```python
from build123d import *

# Parameters (mm, degrees)
SKETCH1_W           = 43.18
SKETCH1_H           = 17.78
BOSS_EXTRUDE1_DEPTH = 12.7
CUT_EXTRUDE1_DEPTH  = 7.62
CUT_EXTRUDE2_DEPTH  = 18.78


with BuildPart() as part:
    # Sketch1 → Boss-Extrude1 (new body)
    with BuildSketch(Plane.XY):
        with Locations((21.59, 8.89)):
            Rectangle(SKETCH1_W, SKETCH1_H)
    extrude(amount=-BOSS_EXTRUDE1_DEPTH)

    # Sketch3 → Cut-Extrude1 (cut)
    with BuildSketch(Plane(origin=(0, 17.78, 0), x_dir=(1, 0, 0), z_dir=(0, 1, 0))):
        Polygon((43.18, 12.7), (36.83, 6.35), (43.18, 0), align=None)
    extrude(amount=-CUT_EXTRUDE1_DEPTH, mode=Mode.SUBTRACT)

    # Sketch4 → Cut-Extrude2 (cut, through all)
    with BuildSketch(Plane(origin=(0, 17.78, 0), x_dir=(1, 0, 0), z_dir=(0, 1, 0))):
        with BuildLine():
            Line((32.381000008, 4.599999944), (24.260999992, 4.599999944))
            ThreePointArc((24.260999992, 4.599999944), (22.510999936, 6.35), (24.260999992, 8.100000056))
            Line((24.260999992, 8.100000056), (32.381000008, 8.100000056))
            ThreePointArc((32.381000008, 8.100000056), (34.131000064, 6.35), (32.381000008, 4.599999944))
        make_face()
        with BuildLine():
            Line((15.68099988, 4.599999944), (7.560999864, 4.599999944))
            ThreePointArc((7.560999864, 4.599999944), (5.810999808, 6.35), (7.560999864, 8.100000056))
            Line((7.560999864, 8.100000056), (15.68099988, 8.100000056))
            ThreePointArc((15.68099988, 8.100000056), (17.430999936, 6.35), (15.68099988, 4.599999944))
        make_face()
    extrude(amount=-CUT_EXTRUDE2_DEPTH, mode=Mode.SUBTRACT)


solid = part.part
```
Design review of the part built by this model. Coordinates are the model's own, in mm. A direction names the side the tool comes from. Coordinates: 2 decimals unless noted, no trailing zeros. Order: outer loops, then holes, each group sorted by start corner. A loop starts at its lowest first (then second) coordinate and runs counter-clockwise, first axis right, second up. Notation, with made-up numbers: M 58.25,46 L 72.25,46 A15 ccw 72.25,74 Z; hole C -19.75,19 d3. An arc over 180 degrees is marked long. Answer as a JSON object with one key per item and string values. Group by question number.
1) Mouldability with a two-part tool opening along X and no side actions: class faces 1 (the flat face through (0, 9, -6)), 2 (the flat face through (12, 9, -4.6)), 3 (the flat face through (41, 10.16, -6)), 4 (the flat face through (40.05, 14.02, -9.57)) as pulls with the +X half, pulls with the -X half, needs draft (parallel to the pull), parting line crosses it, or undercut.
2) Wall thickness on L1, parallel to Z at x = 11.5, y = 8.25; L2, parallel to X at y = 10.25, z = -7.5; L3, parallel to X at y = 10.75, z = -5.25: over which ranges is each line inside the solid? List them lowest first.
3) Tool access review of faces 5 (the flat face through (21, 17.78, -6)), 6 (the flat face through (39.96, 14.02, -3.22)), 7 (the flat face through (28, 9, -4.6)): name each direction out of +Z, -Z, +X, -X, +Y, -Y from which nothing blocks a thin tool from reaching the whole face with its end or side.
4) For pin 1 (6 mm diameter, centred on y = 14, z = -10.5, fed in from +X), flat-tipped, find the tip position at first contact; note if it passes through.
5) Add section A-A, the plane x = 15. Write out the cut boundary in (y, z), then the cut area to 3 significant figures.
6) Add section C-C, the plane y = 11.75. Write out the cut boundary in (x, z).
7) Add section B-B, the plane z = -6.75. Write out the cut boundary in (x, y).
8) Add section D-D, the plane z = -9. Write out the cut boundary in (x, y), then the cut area to 3 significant figures.
Computed values:
{
 "1": {"face 1": "pulls with the -X half", "face 2": "undercut", "face 3": "needs draft", "face 4": "pulls with the +X half"},
 "2": {"L1": "z = -12.7 to -8.1, -4.6 to 0", "L2": "x = 0 to 6.24, 17 to 22.94, 33.7 to 37.98", "L3": "x = 0 to 6.2, 17.04 to 22.9, 33.74 to 37.93"},
 "3": {"face 5": "+Z, -Z, +X, -X, +Y", "face 6": "+X, +Y", "face 7": "+Y, -Y"},
 "4": {"pin 1": "stops at x = 43.18"},
 "5": {"outline": "M 0,-12.7 L 17.78,-12.7 L 17.78,-8.1 L 0,-8.1 Z; M 0,-4.6 L 17.78,-4.6 L 17.78,0 L 0,0 Z", "area": "164 mm^2"},
 "6": {"outline": "M 0,-12.7 L 43.18,-12.7 L 36.83,-6.35 L 43.18,0 L 0,0 Z; hole M 7.56,-8.1 L 15.68,-8.1 A1.75 ccw 15.68,-4.6 L 7.56,-4.6 A1.75 ccw Z; hole M 24.26,-8.1 L 32.38,-8.1 A1.75 ccw 32.38,-4.6 L 24.26,-4.6 A1.75 ccw Z"},
 "7": {"outline": "M 0,0 L 5.86,0 L 5.86,17.78 L 0,17.78 Z; M 17.38,0 L 22.56,0 L 22.56,17.78 L 17.38,17.78 Z; M 34.08,0 L 43.18,0 L 43.18,10.16 L 37.23,10.16 L 37.23,17.78 L 34.08,17.78 Z"},
 "8": {"outline": "M 0,0 L 43.18,0 L 43.18,10.16 L 39.48,10.16 L 39.48,17.78 L 0,17.78 Z", "area": "740 mm^2"}
}
